Autodesk Inventor part; units mm, degrees
ref_plane "YZ Plane" through (0, 0, 0) normal (1, 0, 0) x (0, 1, 0)
ref_plane "XZ Plane" through (0, 0, 0) normal (0, 1, 0) x (-1, 0, 0)
ref_plane "XY Plane" through (0, 0, 0) normal (0, 0, 1) x (1, 0, 0)
sketch "Skizze1" plane through (0, 0, 0) normal (0, 0, 1) x (1, 0, 0)
  circle A0 centre (0, 0) radius 5.95
  dimension "d0" = 11.9
extrude "Extrusion1" add sketch "Skizze1" along normal blind 2.55
sketch "Skizze2" plane through (0, 0, 2.55) normal (0, 0, 1) x (1, 0, 0)
  circle A0 centre (0, 0) radius 6.95
  circle A1 centre (0, 0) radius 5.95
  dimension "d5" = 1
extrude "Extrusion2" add sketch "Skizze2" along normal blind 2 contours A0 | A1
mirror "Spiegeln1" about plane through (0, 0, 0) normal (0, 0, -1) of "Extrusion2", "Extrusion1"
sketch "Skizze3" plane through (0, 0, 4.55) normal (0, 0, 1) x (1, 0, 0)
  point P0 (0, 0)
  point P1 (0, 0)
hole "Bohrung1" at (0, 0, 4.55) direction (0, 0, -1) diameter 6 end through all counterbore diameter 11.2 counterbore depth 2
chamfer "Fasen1" distance 1 angle 45 1 edges at (-6.95, 0, 2.55)
properties part number "SolarPlugAdapter"
Here's how the part is built. I have some questions about the finished solid (model axes, mm). A direction names the side the tool comes from. Coordinates: 2 decimals unless noted, no trailing zeros. Order: outer loops, then holes, each group sorted by start corner. A loop starts at its lowest first (then second) coordinate and runs counter-clockwise, first axis right, second up. Notation, with made-up numbers: (83.25, -18.75) -> (126.25, -18.75) arc R14 ccw to (126.25, -0.75) -> close; hole circle Ø2 at (-4, -20.5). An arc over 180 degrees is marked (long way). Return JSON: item names as keys, results as strings.
1) I'm going to push flat-ended pins straight in: P1, Ø1, axis at x = 3.5, z = -2, coming from the -Y side; P2, Ø1, axis at x = 0, z = 2.5, coming from the +Y side; P3, Ø4, axis at x = 3.5, y = -0.5, coming from the +Z side. Where does each tip first touch, or does it pass through?
Conclusion:
{"P1": "stops at y = -5.14", "P2": "stops at y = 6.4", "P3": "stops at z = 2.55"}
2) Thinking about a two-plate mould opening in Y: for faces 4 (the flat face through (-1, -3, -4.55)), 5 (the flat face through (2.4, -2.4, 2.55)), 6 (the cylindrical face through (-4.385, 4.021, 0.036)), which applies, +Y half, -Y half, draft (parallel to the pull), parting line (faces both ways), or undercut?
Conclusion:
{"face 4": "draft", "face 5": "undercut", "face 6": "parting line"}
3) On a 3-axis mill with a long thin cutter (end or side, diameter ignored), from which of +Z, -Z, +X, -X, +Y, -Y can I reach the whole of each face in a straight line? I mean faces 1 (the flat face through (-5, 3, 4.55)), 2 (the flat face through (-6, 2, -2.55)), 3 (the cylindrical face through (-0.246, 5.595, 3.536)). Say none if no direction works.
Conclusion:
{"face 1": "+Z, +X, -X, +Y, -Y", "face 2": "none", "face 3": "+Z"}
4) If we section it at D-D on z = 3.25: List the corners of the cut face in (x, y) for me, plus the area to 3 significant figures.
Conclusion:
{"outline": "circle Ø13.3 at (0, 0); hole circle Ø11.2 at (0, 0)", "area": "40.4 mm²"}
5) If I drill on probe 1 along Y at (x, z) = (0, 1.25); probe 2 along Z at (x, y) = (2.5, -3.75); probe 3 along Y at (x, z) = (0.5, -3.5), over which ranges is the centre line in solid material (lowest first)?
Conclusion:
{"probe 1": "y = -5.95 to -3, 3 to 5.95", "probe 2": "z = -4.55 to 2.55", "probe 3": "y = -6.93 to -2.96, 2.96 to 6.93"}
6) If we section it at C-C on z = -1: List the corners of the cut face in (x, y) for me.
Conclusion:
{"outline": "circle Ø11.9 at (0, 0); hole circle Ø6 at (0, 0)"}
